```python
from build123d import *

# Parameters (mm, degrees)
ESBO_O1_R                = 10
RESSALTO_EXTRUS_O1_DEPTH = 4.25
RESSALTO_EXTRUS_O2_START = 3
ESBO_O2_R                = 10
RESSALTO_EXTRUS_O2_DEPTH = 3
CORTE_EXTRUS_O1_REACH    = 17.892
ESBO_O3_R                = 1.5
ESBO_O5_R                = 6
CORTE_EXTRUS_O3_DEPTH    = 2.5


with BuildPart() as part:
    # Esboço1 → Ressalto-extrusão1 (new body)
    with BuildSketch(Plane(origin=(0, 0, 0), x_dir=(0, 0, -1), z_dir=(1, 0, 0))):
        Circle(ESBO_O1_R)
    extrude(amount=RESSALTO_EXTRUS_O1_DEPTH)

    # Esboço2 → Ressalto-extrusão2 (add)
    with BuildSketch(Plane.ZY.offset(RESSALTO_EXTRUS_O2_START)):
        Circle(ESBO_O2_R)
    extrude(amount=-RESSALTO_EXTRUS_O2_DEPTH)

    # Esboço3 → Corte-extrusão1 (cut, up to next)
    with BuildSketch(Plane(origin=(4.25, 0, 0), x_dir=(0, 0, -1), z_dir=(1, 0, 0)), mode=Mode.PRIVATE) as corte_extrus_o1_sk1:
        Circle(ESBO_O3_R)
    corte_extrus_o1_tool1 = extrude(corte_extrus_o1_sk1.sketch, amount=-CORTE_EXTRUS_O1_REACH, mode=Mode.PRIVATE) & part.part
    add(corte_extrus_o1_tool1.solids().sort_by_distance((4.25, 0, 0))[0], mode=Mode.SUBTRACT)

    # Esboço5 → Corte-extrusão3 (cut)
    with BuildSketch(Plane.ZY.offset(3)):
        Circle(ESBO_O5_R)
    extrude(amount=-CORTE_EXTRUS_O3_DEPTH, mode=Mode.SUBTRACT)


solid = part.part
```
Geometry: final body of the model. Coordinates: model frame, mm. A direction names the side the tool comes from. Round coordinates to 2 decimals unless told otherwise and drop trailing zeros. Order: outer loops, then holes, each group sorted by start corner. A loop starts at its lowest first (then second) coordinate and runs counter-clockwise, first axis right, second up. Notation, with made-up numbers: M 59.25,-35.75 L 113.25,-35.75 A16 cw 113.25,-20.75 Z; hole C 2.5,61.25 d3. An arc over 180 degrees is marked long. One line per item, written item: value.
(1) Pin query (flat end, axial travel): P1, Ø1.5, axis at x = 2.5, z = -4, coming from the +Y side. Return the tip coordinate at first contact, or that it passes through.
Result sheet:
P1: y = 9.46
(2) Cut plane C-C (x = 2.25). Return the cut outline in (y, z), and give its area (3 significant figures).
Result sheet:
outline: C 0,0 d20; hole C 0,0 d3
area: 307 mm2
(3) Cut plane A-A (y = 0). Return the cut outline in (x, z).
Result sheet:
outline: M -3,-10 L 4.25,-10 L 4.25,-1.5 L -0.5,-1.5 L -0.5,-6 L -3,-6 Z; M -3,6 L -0.5,6 L -0.5,1.5 L 4.25,1.5 L 4.25,10 L -3,10 Z
(4) Pull-direction query (Y, two-part tool) for faces 3 (the cylindrical face through (1.91, 0.07, 1.5)), 4 (the flat face through (-3, -7, 0)); classes: pulls with the +Y half, pulls with the -Y half, needs draft (parallel to the pull), parting line crosses it, or undercut.
Result sheet:
face 3: undercut
face 4: needs draft
(5) Line query: probe 1 along Y at (x, z) = (0.6, 0); probe 2 along Y at (x, z) = (-2.4, 0); probe 3 along X at (y, z) = (-0.25, 3.5). Output: solid intervals per line, ascending. Write a range as [from, to].
Result sheet:
probe 1: [-10, -1.5], [1.5, 10]
probe 2: [-10, -6], [6, 10]
probe 3: [-0.5, 4.25]
(6) Reachability of faces 1 (the flat face through (4.25, 0, -2)), 2 (the cylindrical face through (-2, 0, -6)) from +Z, -Z, +X, -X, +Y, -Y: full face, straight path, thin tool, end or side. Return the list, or none.
Result sheet:
face 1: +Z, -Z, +X, +Y, -Y
face 2: -X
(7) Cut plane D-D (y = -4.5). Return the cut outline in (x, z), and give its area (3 significant figures).
Result sheet:
outline: M -3,-8.93 L 4.25,-8.93 L 4.25,8.93 L -3,8.93 L -3,3.97 L -0.5,3.97 L -0.5,-3.97 L -3,-3.97 Z
area: 110 mm2
